Check sheet for the drawn part. Datum: minimum x, y, z corner. Units: mm. A direction names the side the tool comes from. Round coordinates to 2 decimals unless told otherwise and drop trailing zeros. Write each loop counter-clockwise with the first axis right and the second up, starting at its lowest first coordinate (ties: lowest second). Pieces come first, ordered by that corner, then holes. Notation, with made-up numbers: (-16, -6) -> (7, -6) arc R25 cw to (7, 8) -> close; hole circle Ø8 at (1, 82.5). An arc over 180 degrees is marked (long way). Use a Markdown table: item, result.
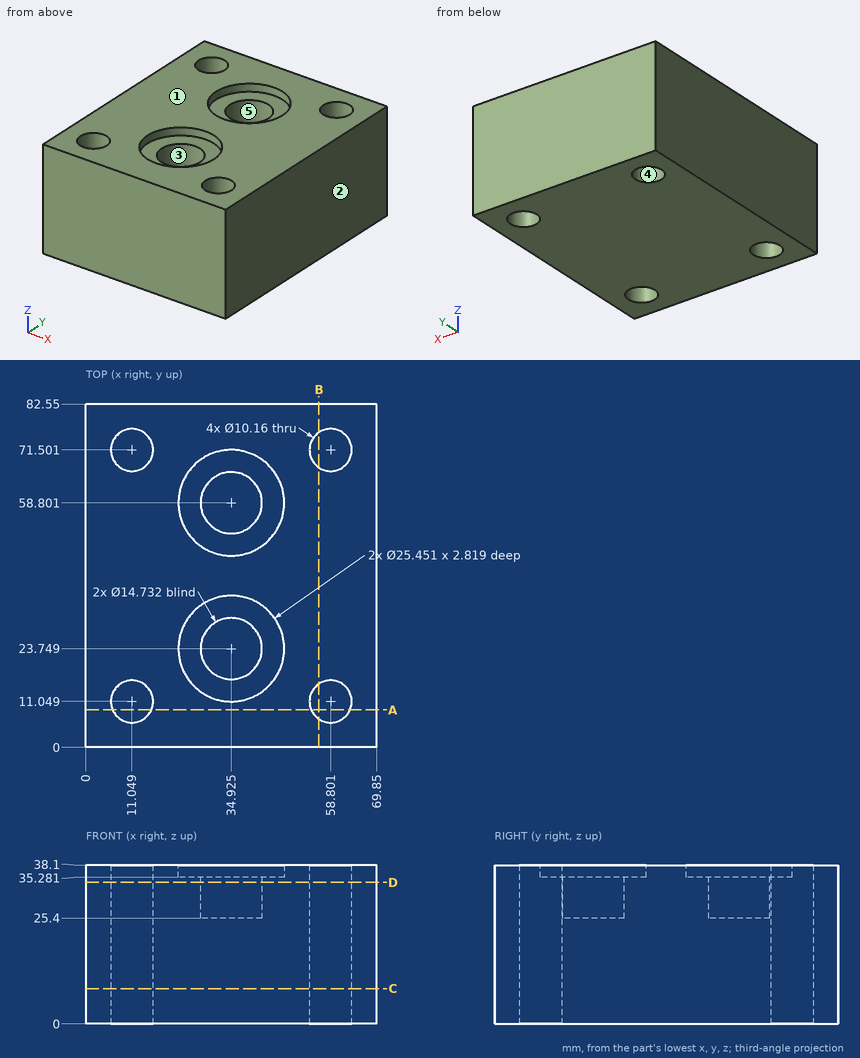
(1) Release check for a two-part mould opening along X. For the marked faces 1, 2 and 3 record: +X half, -X half, draft (parallel to the pull), parting line (faces both ways), or undercut.
A:
| item | result |
|---|---|
| face 1 | draft |
| face 2 | +X half |
| face 3 | undercut |
(2) Section check D-D on z = 34. State how many separate pieces and enclosed holes the cut face has, plus the area to 3 significant figures.
A:
| item | result |
|---|---|
| separate pieces | 1 |
| enclosed holes | 6 |
| area | 5,100 mm2 |
(3) Section check B-B on x = 56. Record the cut outline in (y, z).
A:
| item | result |
|---|---|
| outline | (0, 0) -> (6.81, 0) -> (6.81, 38.1) -> (0, 38.1) -> close; (15.29, 0) -> (67.26, 0) -> (67.26, 38.1) -> (15.29, 38.1) -> close; (75.74, 0) -> (82.55, 0) -> (82.55, 38.1) -> (75.74, 38.1) -> close |
(4) Gauge pin test, flat ends, axial feed: pin 1 Ø12 at (x, y) = (34.925, 58.801) entering from +Z; pin 2 Ø16.5 at (x, y) = (58.801, 71.501) entering from -Z; pin 3 Ø12 at (x, y) = (31.5, 62) entering from +Z. Record the tip position at first contact, or that the pin passes through.
A:
| item | result |
|---|---|
| pin 1 | stops at z = 25.4 |
| pin 2 | stops at z = 0 |
| pin 3 | stops at z = 35.28 |
(5) Thickness scan on line 1 (Y direction, x = 11, z = 26); line 2 (X direction, y = 9, z = 24.5); line 3 (Y direction, x = 55, z = 30). Record the ranges inside material, lowest first.
A:
| item | result |
|---|---|
| line 1 | y = 0 to 5.97, 16.13 to 66.42, 76.58 to 82.55 |
| line 2 | x = 0 to 6.4, 15.7 to 54.15, 63.45 to 69.85 |
| line 3 | y = 0 to 7.68, 14.42 to 68.13, 74.87 to 82.55 |
(6) Access from +Z, -Z, +X, -X, +Y, -Y to the whole of each face (thin tool, end or side, straight path). Record for the marked faces 4 and 5.
A:
| item | result |
|---|---|
| face 4 | +Z, -Z |
| face 5 | +Z |
(7) Section check A-A on y = 9. Record the cut outline in (x, z), plus the area to 3 significant figures.
A:
| item | result |
|---|---|
| outline | (0, 0) -> (6.4, 0) -> (6.4, 38.1) -> (0, 38.1) -> close; (15.7, 0) -> (54.15, 0) -> (54.15, 38.1) -> (15.7, 38.1) -> close; (63.45, 0) -> (69.85, 0) -> (69.85, 38.1) -> (63.45, 38.1) -> close |
| area | 1,950 mm2 |
(8) Section check C-C on z = 8.5. Record the cut outline in (x, y).
A:
| item | result |
|---|---|
| outline | (0, 0) -> (69.85, 0) -> (69.85, 82.55) -> (0, 82.55) -> close; hole circle Ø10.16 at (11.05, 11.05); hole circle Ø10.16 at (11.05, 71.5); hole circle Ø10.16 at (58.8, 11.05); hole circle Ø10.16 at (58.8, 71.5) |
